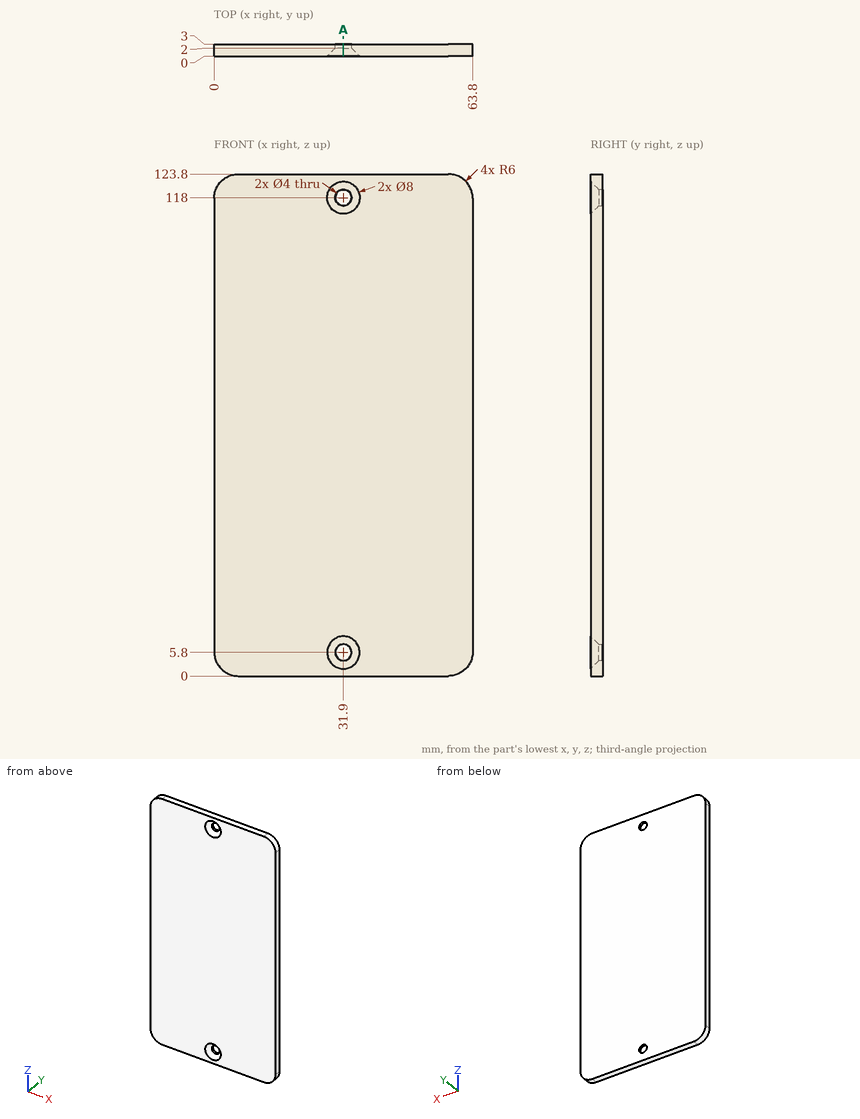
The figure shows three views and two pictorial views of one solid part (mm, origin at its lowest corner). Answer the questions. Give positions to 0.01 mm unless a question says otherwise; leave off trailing zeros. Write each loop counter-clockwise with the first axis right and the second up, starting at its lowest first coordinate (ties: lowest second). Pieces come first, ordered by that corner, then holes. Notation, with made-up numbers: M -31,17.5 L 19,17.5 A15 ccw 19,31.5 Z; hole C 41.5,75.25 d2. An arc over 180 degrees is marked long. One line per item, written item: value. Start each with the question number.
(1) Find section A-A (x = 31.9). Determine the outline of the cut face in (y, z).
(2) Find the intervals of material crossed by line 1 (Z direction, x = 31.9, y = 2.8); line 2 (X direction, y = 2.75, z = 118); line 3 (Z direction, x = 29.5, y = 1.35), in increasing order.
(3) A flat-ended cylindrical pin translates along its axis: pin 1 Ø3.5 at (x, z) = (31.9, 118) entering from -Y. Find the tip coordinate at first contact, or state that the pin passes through.
Results below:
1. outline: M 0,0 L 3,0 L 3,3.8 L 2,3.8 L 0,1.8 Z; M 0,9.8 L 2,7.8 L 3,7.8 L 3,116 L 2,116 L 0,114 Z; M 0,122 L 2,120 L 3,120 L 3,123.8 L 0,123.8 Z
2. line 1: z = 0 to 3.8, 7.8 to 116, 120 to 123.8
2. line 2: x = 0 to 29.9, 33.9 to 63.8
2. line 3: z = 0 to 4.68, 6.92 to 116.88, 119.12 to 123.8
3. pin 1: passes through
